The listing builds one solid part. Answer for the finished solid, in the listing's coordinates (mm). A direction names the side the tool comes from. Coordinates: 2 decimals unless noted, no trailing zeros. Order: outer loops, then holes, each group sorted by start corner. A loop starts at its lowest first (then second) coordinate and runs counter-clockwise, first axis right, second up. Notation, with made-up numbers: (-23.75, -23.75) -> (7.25, -23.75) arc R10 ccw to (7.25, -19.75) -> close; hole circle Ø5 at (31.5, 67.25). An arc over 180 degrees is marked (long way). Answer in a Markdown table with one row per item.
Autodesk Inventor part; units mm, degrees
ref_plane "Work Plane2" through (2.032, 0, 0) normal (0, 1, 0) x (1, 0, 0)
ref_plane "YZ Plane" through (0, 0, 0) normal (1, 0, 0) x (0, 1, 0)
ref_plane "XZ Plane" through (0, 0, 0) normal (0, 1, 0) x (-1, 0, 0)
sketch "Sketch1" plane through (0, 0, 0) normal (0, 0, 1) x (1, 0, 0)
  line L0 (2.2606, 0) -> (7.9375, 0)
  line L1 (7.9375, 0) -> (7.9375, 1.4224)
  line L2 (7.9375, 1.4224) -> (1.7018, 1.4224)
  line L3 (0.4892, 2.4765) -> (0, 2.4765)
  line L4 (-1.5875, 0) -> (9.525, 0)
  line L5 (0, -0.4953) -> (0, 2.9718)
  line L6 (0, 1.6256) -> (1.8999, 0.6783)
  line L7 (1.8999, 0.6783) -> (2.2606, 0)
  line L8 (1.7018, 1.4224) -> (0.4892, 2.4765)
  line L9 (0, 2.4765) -> (0, 1.6256)
  dimension "d2" = 2.8448
  dimension "d3" = 4.953
  dimension "d4" = 2.2606
  dimension "d5" = 3.2512
  dimension "d6" = 26.5
  dimension "d7" = 62
  dimension "d13" = 41
  dimension "d14" = 1.7018
  dimension "d15" = 7.9375
revolve "Body" add sketch "Sketch1" angle 360 about axis through (2.2606, 0, 0) along (1, 0, 0) contours L7 L6 L5 L3 L8 L2 L1 L0
sketch "Sketch2" plane through (0, 0, 0) normal (-1, 0, 0) x (0, 0, 1)
  line L0 (0, -3.4671) -> (0, 3.4671)
  line L1 (-3.4671, 0) -> (3.4671, 0)
  line L2 (0, 1.6256) -> (0, 0) construction
  line L3 (0, 0) -> (1.6256, 0) construction
  arc A0 (0.5419, 0) -> (0, 0.5419) centre (0, 0) ccw
  line L4 (0, 0) -> (0.7947, 0.7947) construction
  arc A1 (0.8128, 0) -> (0, 0.8128) centre (0, 0) ccw construction
  line L5 (0.2286, 1.6094) -> (0.2202, 0.7824)
  line L6 (1.6094, 0.2286) -> (0.7824, 0.2202)
  arc A2 (0.2202, 0.7824) -> (0.7824, 0.2202) centre (0.7767, 0.7767) ccw
  arc A3 (1.6256, 0) -> (1.6094, 0.2286) centre (0, 0) ccw
  arc A4 (0.2286, 1.6094) -> (0, 1.6256) centre (0, 0) ccw
  arc A5 (1.6094, 0.2286) -> (0.2286, 1.6094) centre (0, 0) ccw
  line L7 (0.2286, -1.6094) -> (0.2202, -0.7824)
  line L8 (1.6094, -0.2286) -> (0.7824, -0.2202)
  arc A6 (0.7824, -0.2202) -> (0.2202, -0.7824) centre (0.7767, -0.7767) ccw
  arc A7 (1.6094, -0.2286) -> (1.6256, 0) centre (0, 0) ccw
  arc A8 (0, -1.6256) -> (0.2286, -1.6094) centre (0, 0) ccw
  arc A9 (0.2286, -1.6094) -> (1.6094, -0.2286) centre (0, 0) ccw
  line L9 (-0.2286, 1.6094) -> (-0.2202, 0.7824)
  line L10 (-1.6094, 0.2286) -> (-0.7824, 0.2202)
  arc A10 (-0.7824, 0.2202) -> (-0.2202, 0.7824) centre (-0.7767, 0.7767) ccw
  arc A11 (-1.6094, 0.2286) -> (-1.6256, 0) centre (0, 0) ccw
  arc A12 (0, 1.6256) -> (-0.2286, 1.6094) centre (0, 0) ccw
  arc A13 (-0.2286, 1.6094) -> (-1.6094, 0.2286) centre (0, 0) ccw
  arc A14 (-1.6094, -0.2286) -> (-0.2286, -1.6094) centre (0, 0) ccw
  arc A15 (-0.2286, -1.6094) -> (0, -1.6256) centre (0, 0) ccw
  arc A16 (-1.6256, 0) -> (-1.6094, -0.2286) centre (0, 0) ccw
  line L11 (-1.6094, -0.2286) -> (-0.7824, -0.2202)
  arc A17 (-0.2202, -0.7824) -> (-0.7824, -0.2202) centre (-0.7767, -0.7767) ccw
  line L12 (-0.2286, -1.6094) -> (-0.2202, -0.7824)
  dimension "d18" = 45
  dimension "d19" = 1.0837
  dimension "d20" = 1.6256
  dimension "d21" = 3.2512
  dimension "d22" = 0.2286
extrude "Slot" add sketch "Sketch2" against normal up to next contours A2 L5 A5 L6 | L9 A10 L10 A13 | L7 A6 L8 A9 | A14 L11 A17 L12
fillet "Fillet1" radius 0.0914 4 edges at (0, 1.6256, 0) (0, 0, 1.6256) (0, -1.6256, 0) (0, 0, -1.6256)
thread "Thread"
chamfer "Chamfer1" distance 0.4763 distance2 0.4763 1 edges at (7.9375, -1.4224, 0) measured on face at (7.9375, -0.0186, 0.3144)
ref_plane "Work Plane2" through (2.032, 0, 0) normal (0, 1, 0) x (1, 0, 0)
equation "\"d2\" = GD"
equation "\"d3\" = KOD"
equation "\"d4\" = INTI"
equation "\"d5\" = SDM"
equation "\"d13\" = 0.5 * SEWI"
equation "\"d14\" = KOH"
equation "\"d15\" = NLG"
equation "\"d19\" = 0.333333 * SDM"
equation "\"d20\" = 0.5 * SDM"
equation "\"d21\" = SDM"
equation "\"d22\" = 0.5 * SBR"
equation "\"d45\" = INTI"
equation "\"d25\" = 0.2 * SBR"
equation "\"d9\" = GEL"
equation "\"d11\" = -0.5 * SPD + 0.5 * GD"
equation "\"d12\" = GUL"
equation "\"GD\" = NND"
equation "\"NLG\" = 7.9375"
equation "\"GEL\" = 4.6482"
equation "\"KOD\" = 4.953"
equation "\"KOH\" = 1.7018"
equation "\"SDM\" = 3.2512"
equation "\"INTI\" = 2.2606"
equation "\"SBR\" = 0.4572"
equation "\"GUL\" = 0.75 * GAL"
equation "\"SPD\" = 1.8923"
equation "\"SEWI\" = 82deg"
equation "\"d0\" = NLG"
equation "\"d1\" = KOH"
equation "\"d17\" = SDM"
equation "\"TOA\" = 30deg"
equation "\"THREADDIA\" = 2.8448"
equation "\"BDM\" = NND"
equation "\"NND\" = 2.8448"
equation "\"GAL\" = 0.635"
equation "\"GD1\" = SPD"
properties part number "ANSI B18.6.3 - 4-40 x 5/16, CRFCHMSTII(5)" material "Steel, Mild"
(1) Find the intervals of material crossed by line 1 along X through (y, z) = (-0.95, -2.15); line 2 along Z through (x, y) = (5.5, -0.05); line 3 along X through (y, z) = (0.15, 0.5), in increasing order. Write a range as from..to.
Check values:
| item | result |
|---|---|
| line 1 | 0..0.63 |
| line 2 | -1.42..1.42 |
| line 3 | 1.98..7.94 |
(2) Flat-ended cylindrical pins translate along their axes: pin 1 (1.5 mm diameter, centred on x = 3.5, z = -0.5, fed in from -Y); pin 2 (1.5 mm diameter, centred on x = 1.5, y = -0.5, fed in from +Z). Find the tip coordinate at first contact, or state that the pin passes through.
Check values:
| item | result |
|---|---|
| pin 1 | y = -1.42 |
| pin 2 | z = 2.21 |
(3) Which of the six approach directions +Z, -Z, +X, -X, +Y, -Y give full straight-line access (tool end or side, diameter ignored) to faces 4 (the flat face through (0, 1, -1)), 5 (the conical face through (1.17, 0.01, -1.04))?
Check values:
| item | result |
|---|---|
| face 4 | +Z, -Z, -X, +Y, -Y |
| face 5 | -X |
(4) For a pull along Y with two mould halves and no side action, classify faces 1 (the conical face through (2.198, 0.109, 0.045)), 2 (the flat face through (7.938, 0, 0)), 3 (the cylindrical face through (4.54, -0.31, 1.39)) as released by +Y, released by -Y, zero draft, split by the parting line, or undercut.
Check values:
| item | result |
|---|---|
| face 1 | undercut |
| face 2 | zero draft |
| face 3 | split by the parting line |
(5) A cutting plane is placed at A-A, the plane x = 4.5. Determine the outline of the cut face in (y, z), then the cut area to 3 significant figures.
Check values:
| item | result |
|---|---|
| outline | circle Ø2.84 at (0, 0) |
| area | 6.36 mm² |
